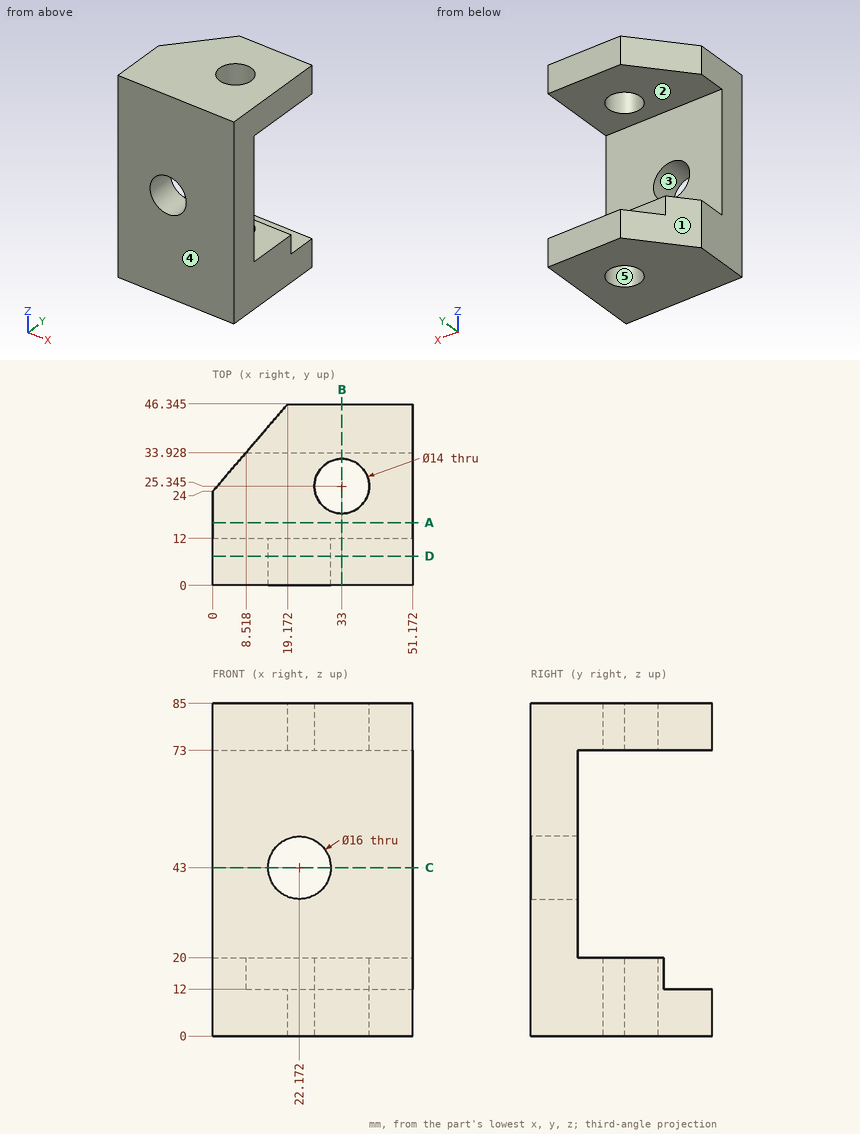
The figure shows three views and two pictorial views of one solid part (mm, origin at its lowest corner). Answer the questions. A direction names the side the tool comes from. Coordinates: 2 decimals unless noted, no trailing zeros. Write each loop counter-clockwise with the first axis right and the second up, starting at its lowest first coordinate (ties: lowest second). Pieces come first, ordered by that corner, then holes.
1. Flat-ended cylindrical pins translate along their axes: pin 1 (8.5 mm diameter, centred on x = 33, y = 25.34, fed in from +Z); pin 2 (12 mm diameter, centred on x = 23.5, z = 27, fed in from +Y). Find the tip coordinate at first contact, or state that the pin passes through.
Results list:
pin 1: passes through
pin 2: stops at y = 12
2. Consider line 1 along Z through (x, y) = (48, 26); line 2 along Z through (x, y) = (39.5, 39); line 3 along Y through (x, z) = (33, 77.25) (1 decimal). Determine where each line is inside the solid, lowest interval first.
Results list:
line 1: z = 0 to 20, 73 to 85
line 2: z = 0 to 12, 73 to 85
line 3: y = 0 to 18.3, 32.3 to 46.3
3. The part is cut by section D-D, the plane y = 7.5. Write down the section's boundary in (x, z), and give its area (3 significant figures).
Results list:
outline: (0, 0) - (51.17, 0) - (51.17, 85) - (0, 85) - close; hole circle Ø16 at (22.17, 43)
area: 4,150 mm2
4. The part is cut by section C-C, the plane z = 43. Write down the section's boundary in (x, y), and give its area (3 significant figures).
Results list:
outline: (0, 0) - (14.17, 0) - (14.17, 12) - (0, 12) - close; (30.17, 0) - (51.17, 0) - (51.17, 12) - (30.17, 12) - close
area: 422 mm2
5. The part is cut by section B-B, the plane x = 33. Write down the section's boundary in (y, z) (1 decimal).
Results list:
outline: (0, 0) - (18.3, 0) - (18.3, 20) - (12, 20) - (12, 73) - (18.3, 73) - (18.3, 85) - (0, 85) - close; (32.3, 0) - (46.3, 0) - (46.3, 12) - (33.9, 12) - (33.9, 20) - (32.3, 20) - close; (32.3, 73) - (46.3, 73) - (46.3, 85) - (32.3, 85) - close
6. The part is cut by section A-A, the plane y = 16. Write down the section's boundary in (x, z), and give its area (3 significant figures).
Results list:
outline: (0, 0) - (51.17, 0) - (51.17, 20) - (0, 20) - close; (0, 73) - (51.17, 73) - (51.17, 85) - (0, 85) - close
area: 1,640 mm2
7. For the marked faces 1 and 2, determine the directions among +Z, -Z, +X, -X, +Y, -Y from which every point of the face is accessible in a straight line to the end or side of a thin tool.
Results list:
face 1: +Z, -Z, -X, +Y
face 2: +X, -X, +Y
8. For a pull along Y with two mould halves and no side action, classify the marked faces 3, 4 and 5 as +Y half, -Y half, draft (parallel to the pull), parting line (faces both ways), or undercut.
Results list:
face 3: draft
face 4: -Y half
face 5: undercut
